Build history of the part. All positions in model axes, mm. A direction names the side the tool comes from. Give positions to 0.01 mm unless a question says otherwise; leave off trailing zeros. Order: outer loops, then holes, each group sorted by start corner. A loop starts at its lowest first (then second) coordinate and runs counter-clockwise, first axis right, second up. Notation, with made-up numbers: (-2.5, 0) - (52.5, 0) arc R35 cw to (52.5, 32) - close; hole circle Ø8 at (74.5, 46). An arc over 180 degrees is marked (long way). One line per item, written item: value.
```python
from build123d import *

# Parameters (mm, degrees)
BOSS_EXTRUDE1_DEPTH = 0.6
BOSS_EXTRUDE2_DEPTH = 1.5
FILLET1_R           = 1


with BuildPart() as part:
    # Sketch2 → Boss-Extrude1 (new body)
    with BuildSketch(Plane.XY):
        Polygon((-9, 11), (-4.4, 11), (-4.4, 12), (-1.2, 12), (-1.2, 11), (11, 11), (11, 2.5), (-9, 2.5), align=None)
    extrude(amount=-BOSS_EXTRUDE1_DEPTH)

    # Sketch1 → Boss-Extrude2 (add)
    with BuildSketch(Plane.XY):
        with BuildLine():
            add(Edge.make_bspline(
                [(8.5, 7.582250387), (8.448081693, 7.453099482), (8.337951661, 7.179459039), (8.156392198, 6.75959463), (7.928053742, 6.343866223), (7.606398256, 6.024741111), (7.260761425, 5.790247234), (7.028066866, 5.65925749), (6.916719247, 5.6)],
                knots=[0.057904746, 0.057904746, 0.057904746, 0.057904746, 0.169421818, 0.28093889, 0.503973033, 0.727007177, 0.838524249, 0.95004132, 0.95004132, 0.95004132, 0.95004132], degree=3))
            add(Edge.make_bspline(
                [(6.916719247, 5.6), (7.028066866, 5.54074251), (7.260761425, 5.409752766), (7.606398256, 5.175258889), (7.928053742, 4.856133777), (8.156392198, 4.44040537), (8.337951661, 4.020540961), (8.448081693, 3.746900518), (8.5, 3.617749613)],
                knots=[0.057904746, 0.057904746, 0.057904746, 0.057904746, 0.169421818, 0.28093889, 0.503973033, 0.727007177, 0.838524249, 0.95004132, 0.95004132, 0.95004132, 0.95004132], degree=3))
            add(Edge.make_bspline(
                [(8.5, 3.617749613), (8.551918307, 3.746900518), (8.662048339, 4.020540961), (8.843607802, 4.44040537), (9.071946258, 4.856133777), (9.393601744, 5.175258889), (9.739238575, 5.409752766), (9.971933134, 5.54074251), (10.083280753, 5.6)],
                knots=[0.057904746, 0.057904746, 0.057904746, 0.057904746, 0.169421818, 0.28093889, 0.503973033, 0.727007177, 0.838524249, 0.95004132, 0.95004132, 0.95004132, 0.95004132], degree=3))
            add(Edge.make_bspline(
                [(10.083280753, 5.6), (9.971933134, 5.65925749), (9.739238575, 5.790247234), (9.393601744, 6.024741111), (9.071946258, 6.343866223), (8.843607802, 6.75959463), (8.662048339, 7.179459039), (8.551918307, 7.453099482), (8.5, 7.582250387)],
                knots=[0.057904746, 0.057904746, 0.057904746, 0.057904746, 0.169421818, 0.28093889, 0.503973033, 0.727007177, 0.838524249, 0.95004132, 0.95004132, 0.95004132, 0.95004132], degree=3))
        make_face()
        with BuildLine():
            add(Edge.make_bspline(
                [(-2.8, 7.617749613), (-2.748081693, 7.746900518), (-2.637951661, 8.020540961), (-2.456392198, 8.44040537), (-2.228053742, 8.856133777), (-1.906398256, 9.175258889), (-1.560761425, 9.409752766), (-1.328066866, 9.54074251), (-1.216719247, 9.6)],
                knots=[0.057904746, 0.057904746, 0.057904746, 0.057904746, 0.169421818, 0.28093889, 0.503973033, 0.727007177, 0.838524249, 0.95004132, 0.95004132, 0.95004132, 0.95004132], degree=3))
            add(Edge.make_bspline(
                [(-1.216719247, 9.6), (-1.328066866, 9.65925749), (-1.560761425, 9.790247234), (-1.906398256, 10.024741111), (-2.228053742, 10.343866223), (-2.456392198, 10.75959463), (-2.637951661, 11.179459039), (-2.748081693, 11.453099482), (-2.8, 11.582250387)],
                knots=[0.057904746, 0.057904746, 0.057904746, 0.057904746, 0.169421818, 0.28093889, 0.503973033, 0.727007177, 0.838524249, 0.95004132, 0.95004132, 0.95004132, 0.95004132], degree=3))
            add(Edge.make_bspline(
                [(-2.8, 11.582250387), (-2.851918307, 11.453099482), (-2.962048339, 11.179459039), (-3.143607802, 10.75959463), (-3.371946258, 10.343866223), (-3.693601744, 10.024741111), (-4.039238575, 9.790247234), (-4.271933134, 9.65925749), (-4.383280753, 9.6)],
                knots=[0.057904746, 0.057904746, 0.057904746, 0.057904746, 0.169421818, 0.28093889, 0.503973033, 0.727007177, 0.838524249, 0.95004132, 0.95004132, 0.95004132, 0.95004132], degree=3))
            add(Edge.make_bspline(
                [(-4.383280753, 9.6), (-4.271933134, 9.54074251), (-4.039238575, 9.409752766), (-3.693601744, 9.175258889), (-3.371946258, 8.856133777), (-3.143607802, 8.44040537), (-2.962048339, 8.020540961), (-2.851918307, 7.746900518), (-2.8, 7.617749613)],
                knots=[0.057904746, 0.057904746, 0.057904746, 0.057904746, 0.169421818, 0.28093889, 0.503973033, 0.727007177, 0.838524249, 0.95004132, 0.95004132, 0.95004132, 0.95004132], degree=3))
        make_face()
        with BuildLine():
            add(Edge.make_bspline(
                [(-6.7, 7.182250387), (-6.751918307, 7.053099482), (-6.862048339, 6.779459039), (-7.043607802, 6.35959463), (-7.271946258, 5.943866223), (-7.593601744, 5.624741111), (-7.939238575, 5.390247234), (-8.171933134, 5.25925749), (-8.283280753, 5.2)],
                knots=[0.057904746, 0.057904746, 0.057904746, 0.057904746, 0.169421818, 0.28093889, 0.503973033, 0.727007177, 0.838524249, 0.95004132, 0.95004132, 0.95004132, 0.95004132], degree=3))
            add(Edge.make_bspline(
                [(-8.283280753, 5.2), (-8.171933134, 5.14074251), (-7.939238575, 5.009752766), (-7.593601744, 4.775258889), (-7.271946258, 4.456133777), (-7.043607802, 4.04040537), (-6.862048339, 3.620540961), (-6.751918307, 3.346900518), (-6.7, 3.217749613)],
                knots=[0.057904746, 0.057904746, 0.057904746, 0.057904746, 0.169421818, 0.28093889, 0.503973033, 0.727007177, 0.838524249, 0.95004132, 0.95004132, 0.95004132, 0.95004132], degree=3))
            add(Edge.make_bspline(
                [(-6.7, 3.217749613), (-6.648081693, 3.346900518), (-6.537951661, 3.620540961), (-6.356392198, 4.04040537), (-6.128053742, 4.456133777), (-5.806398256, 4.775258889), (-5.460761425, 5.009752766), (-5.228066866, 5.14074251), (-5.116719247, 5.2)],
                knots=[0.057904746, 0.057904746, 0.057904746, 0.057904746, 0.169421818, 0.28093889, 0.503973033, 0.727007177, 0.838524249, 0.95004132, 0.95004132, 0.95004132, 0.95004132], degree=3))
            add(Edge.make_bspline(
                [(-5.116719247, 5.2), (-5.228066866, 5.25925749), (-5.460761425, 5.390247234), (-5.806398256, 5.624741111), (-6.128053742, 5.943866223), (-6.356392198, 6.35959463), (-6.537951661, 6.779459039), (-6.648081693, 7.053099482), (-6.7, 7.182250387)],
                knots=[0.057904746, 0.057904746, 0.057904746, 0.057904746, 0.169421818, 0.28093889, 0.503973033, 0.727007177, 0.838524249, 0.95004132, 0.95004132, 0.95004132, 0.95004132], degree=3))
        make_face()
    extrude(amount=BOSS_EXTRUDE2_DEPTH)

    # Fillet1
    fillet1_edges = [part.edges().sort_by_distance(p)[0] for p in [
        (-9, 2.5, -0.3),
        (11, 2.5, -0.3),
        (11, 11, -0.3),
        (-1.2, 12, -0.3),
        (-4.4, 12, -0.3),
        (-9, 11, -0.3),
    ]]
    fillet(fillet1_edges, radius=FILLET1_R - 0.0001)  # a hair under: the kernel refuses the full size


solid = part.part
```
(1) 3-axis set-ups, long thin cutter, end or side, ignore diameter. For faces 1 (the face through (-1.501, 11.715, -0.304)), 2 (the face through (1, 7, 0)): which of +Z, -Z, +X, -X, +Y, -Y reach the whole face in a straight line?
Completed:
face 1: +Z, -Z, +X, +Y
face 2: +Z
(2) Pin check, flat tips, straight feed: P1, Ø1, axis at x = 0, z = 0, coming from the +Y side; P2, Ø1, axis at x = -5, y = 9.5, coming from the +Z side. Stop position of each tip, or through.
Completed:
P1: y = 11
P2: z = 0
(3) Drill centre lines: line 1 (Y direction, x = 9, z = -0.2); line 2 (Z direction, x = 3.5, y = 6.5); line 3 (X direction, y = 5.75, z = 1). Where is each one in solid material? Low to high.
Completed:
line 1: 2.5 to 11
line 2: -0.6 to 0
line 3: -7.48 to -5.92, 7.18 to 9.82
(4) Slice it at C-C, the plane z = 0.85. Count the separate pieces of the cut face and the enclosed holes in it, and give its area (3 significant figures).
Completed:
separate pieces: 3
enclosed holes: 0
area: 13.1 mm²
(5) Slice it at B-B, the plane x = -1. Give the cut face in (y, z), and give its area (3 significant figures).
Completed:
outline: (2.5, -0.6) - (11, -0.6) - (11, 0) - (2.5, 0) - close
area: 5.10 mm²
